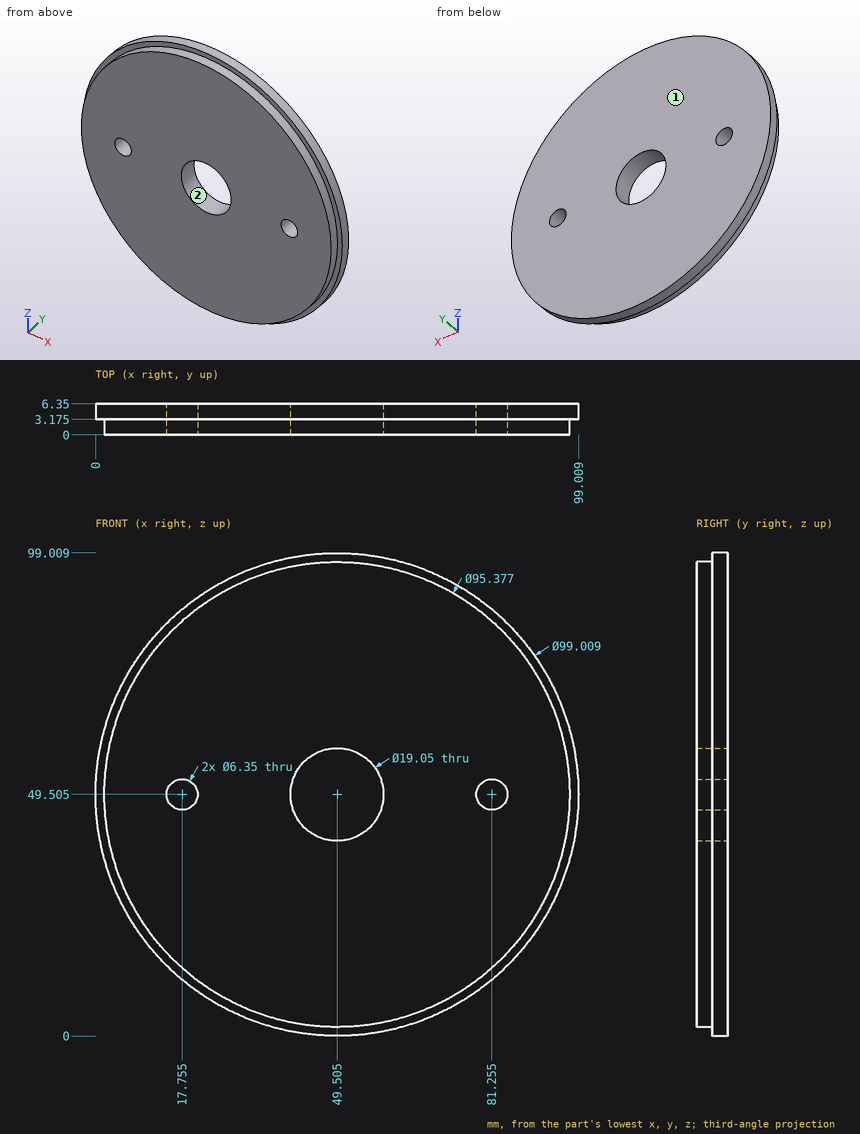
Here's the drawing with two shaded views (mm, measured from the low corner). I have some questions. Give positions to 0.01 mm unless a question says otherwise; leave off trailing zeros. Use a Markdown table: item, result. Add a question column.
Item 1: Will these pins go through, and if not, where does the flat tip stop? pin 1 (3 mm diameter, centred on y = 2.5, z = 52, fed in from +X); pin 2 (2 mm diameter, centred on y = 0.5, z = 85, fed in from -X) (1 decimal); pin 3 (15 mm diameter, centred on x = 49.5, z = 49.5, fed in from -Y).
Item 2: I need wall thicknesses on line 1 (Z direction, x = 80.5, y = 2.5) (1 decimal); line 2 (X direction, y = 6, z = 56.5) (1 decimal); line 3 (Z direction, x = 45, y = 5.75) (1 decimal). Which ranges of each line are inside material? Lowest first, please.
Item 3: If we mould it in two halves opening along Z, with no side actions, what happens to the marked faces 1 and 2? For each: pulls with the +Z half, pulls with the -Z half, needs draft (parallel to the pull), parting line crosses it, or undercut.
Data:
| question | item | result |
|---|---|---|
| 1 | pin 1 | stops at x = 99 |
| 1 | pin 2 | stops at x = 16.6 |
| 1 | pin 3 | passes through |
| 2 | line 1 | z = 13.3 to 46.4, 52.6 to 85.7 |
| 2 | line 2 | x = 0.5 to 43, 56 to 98.5 |
| 2 | line 3 | z = 0.2 to 41.1, 57.9 to 98.8 |
| 3 | face 1 | needs draft |
| 3 | face 2 | undercut |
